Build history of the part. All positions in model axes, mm. A direction names the side the tool comes from. Round coordinates to 2 decimals unless told otherwise and drop trailing zeros. Write each loop counter-clockwise with the first axis right and the second up, starting at its lowest first coordinate (ties: lowest second). Pieces come first, ordered by that corner, then holes. Notation, with made-up numbers: (46.5, 63.5) - (78.5, 63.5) arc R19 ccw to (78.5, 99.5) - close; hole circle Ø7 at (88, -20.5). An arc over 180 degrees is marked (long way). Write each question's results on one line, items separated by ' | '.
from build123d import *

# Parameters (mm, degrees)
F0_W     = 65
F0_H     = 140
F0_W_2   = 9
F0_H_2   = 38
F0_W_3   = 13
F0_H_3   = 14.5
F0_R     = 3.85
F1_DEPTH = 3
F2_DEPTH = 6
F3_DEPTH = 9.5
F4_DEPTH = 13


# Not quite as in the source:
# - a feature names something its author has since deleted; it is built from what else it names


with BuildPart() as f1:
    # F0 (on Top) → F1 (new body)
    with BuildSketch(Plane.XY):
        with Locations((-31.25, -0.0599437952)):
            Rectangle(F0_W, F0_H)
        Polygon((-58.75, -65.0599437952), (-58.75, 64.9400562048), (-3.75, 64.9400562048), (-3.75, 60.4400562048), (-3.75, 49.5400562048), (-3.75, -65.0599437952), align=None, mode=Mode.SUBTRACT)
        Polygon((-3.75, 64.9400562048), (-58.75, 64.9400562048), (-58.75, -65.0599437952), (-3.75, -65.0599437952), (-3.75, 49.5400562048), (-3.75, 60.4400562048), align=None)
        with Locations((-48.45, -37.5599437952)):
            Rectangle(F0_W_2, F0_H_2, mode=Mode.SUBTRACT)
        with Locations((-33.25, -53.8099437952)):
            Rectangle(F0_W_3, F0_H_3, mode=Mode.SUBTRACT)
        with Locations((-33.25, -23.8099437952)):
            Rectangle(F0_W_3, F0_H_3, mode=Mode.SUBTRACT)
        with Locations((-14.75, -38.8099437952)):
            Rectangle(F0_W_3, F0_H_3, mode=Mode.SUBTRACT)
        with Locations((-14.75, -8.8099437952)):
            Rectangle(F0_W_3, F0_H_3, mode=Mode.SUBTRACT)
        with Locations((-48.45, 28.4400562048)):
            Rectangle(F0_W_2, F0_H_2, mode=Mode.SUBTRACT)
        with Locations((-33.25, 6.1900562048)):
            Rectangle(F0_W_3, F0_H_3, mode=Mode.SUBTRACT)
        with Locations((-33.25, 36.1900562048)):
            Rectangle(F0_W_3, F0_H_3, mode=Mode.SUBTRACT)
        with Locations((-14.75, 21.1900562048)):
            Rectangle(F0_W_3, F0_H_3, mode=Mode.SUBTRACT)
        with Locations((-14.75, 51.1900562048)):
            Rectangle(F0_W_3, F0_H_3, mode=Mode.SUBTRACT)
        with Locations((-48.45, 28.4400562048)):
            Rectangle(F0_W_2, F0_H_2)
        with Locations((-48.45, -37.5599437952)):
            Rectangle(F0_W_2, F0_H_2)
        with Locations((-14.75, 51.1900562048)):
            Rectangle(F0_W_3, F0_H_3)
        with Locations((-14.75, 51.1900562048)):
            Circle(F0_R, mode=Mode.SUBTRACT)
        with Locations((-33.25, 36.1900562048)):
            Rectangle(F0_W_3, F0_H_3)
        with Locations((-33.25, 36.1900562048)):
            Circle(F0_R, mode=Mode.SUBTRACT)
        with Locations((-14.75, 21.1900562048)):
            Rectangle(F0_W_3, F0_H_3)
        with Locations((-14.75, 21.1900562048)):
            Circle(F0_R, mode=Mode.SUBTRACT)
        with Locations((-33.25, 6.1900562048)):
            Rectangle(F0_W_3, F0_H_3)
        with Locations((-33.25, 6.1900562048)):
            Circle(F0_R, mode=Mode.SUBTRACT)
        with Locations((-14.75, -8.8099437952)):
            Rectangle(F0_W_3, F0_H_3)
        with Locations((-14.75, -8.8099437952)):
            Circle(F0_R, mode=Mode.SUBTRACT)
        with Locations((-33.25, -23.8099437952)):
            Rectangle(F0_W_3, F0_H_3)
        with Locations((-33.25, -23.8099437952)):
            Circle(F0_R, mode=Mode.SUBTRACT)
        with Locations((-33.25, -53.8099437952)):
            Rectangle(F0_W_3, F0_H_3)
        with Locations((-33.25, -53.8099437952)):
            Circle(F0_R, mode=Mode.SUBTRACT)
        with Locations((-14.75, -38.8099437952)):
            Rectangle(F0_W_3, F0_H_3)
        with Locations((-14.75, -38.8099437952)):
            Circle(F0_R, mode=Mode.SUBTRACT)
    extrude(amount=F1_DEPTH)

    # F0 (on Top) → F2 (join)
    with BuildSketch(Plane.XY):
        with Locations((-31.25, -0.0599437952)):
            Rectangle(F0_W, F0_H)
        Polygon((-58.75, -65.0599437952), (-58.75, 64.9400562048), (-3.75, 64.9400562048), (-3.75, 60.4400562048), (-3.75, 49.5400562048), (-3.75, -65.0599437952), align=None, mode=Mode.SUBTRACT)
        Polygon((-3.75, 64.9400562048), (-58.75, 64.9400562048), (-58.75, -65.0599437952), (-3.75, -65.0599437952), (-3.75, 49.5400562048), (-3.75, 60.4400562048), align=None)
        with Locations((-48.45, -37.5599437952)):
            Rectangle(F0_W_2, F0_H_2, mode=Mode.SUBTRACT)
        with Locations((-33.25, -53.8099437952)):
            Rectangle(F0_W_3, F0_H_3, mode=Mode.SUBTRACT)
        with Locations((-33.25, -23.8099437952)):
            Rectangle(F0_W_3, F0_H_3, mode=Mode.SUBTRACT)
        with Locations((-14.75, -38.8099437952)):
            Rectangle(F0_W_3, F0_H_3, mode=Mode.SUBTRACT)
        with Locations((-14.75, -8.8099437952)):
            Rectangle(F0_W_3, F0_H_3, mode=Mode.SUBTRACT)
        with Locations((-48.45, 28.4400562048)):
            Rectangle(F0_W_2, F0_H_2, mode=Mode.SUBTRACT)
        with Locations((-33.25, 6.1900562048)):
            Rectangle(F0_W_3, F0_H_3, mode=Mode.SUBTRACT)
        with Locations((-33.25, 36.1900562048)):
            Rectangle(F0_W_3, F0_H_3, mode=Mode.SUBTRACT)
        with Locations((-14.75, 21.1900562048)):
            Rectangle(F0_W_3, F0_H_3, mode=Mode.SUBTRACT)
        with Locations((-14.75, 51.1900562048)):
            Rectangle(F0_W_3, F0_H_3, mode=Mode.SUBTRACT)
        with Locations((-48.45, 28.4400562048)):
            Rectangle(F0_W_2, F0_H_2)
        with Locations((-48.45, -37.5599437952)):
            Rectangle(F0_W_2, F0_H_2)
    extrude(amount=F2_DEPTH)

    # F0 (on Top) → F3 (join)
    with BuildSketch(Plane.XY):
        with Locations((-31.25, -0.0599437952)):
            Rectangle(F0_W, F0_H)
        Polygon((-58.75, -65.0599437952), (-58.75, 64.9400562048), (-3.75, 64.9400562048), (-3.75, 60.4400562048), (-3.75, 49.5400562048), (-3.75, -65.0599437952), align=None, mode=Mode.SUBTRACT)
        Polygon((-3.75, 64.9400562048), (-58.75, 64.9400562048), (-58.75, -65.0599437952), (-3.75, -65.0599437952), (-3.75, 49.5400562048), (-3.75, 60.4400562048), align=None)
        with Locations((-48.45, -37.5599437952)):
            Rectangle(F0_W_2, F0_H_2, mode=Mode.SUBTRACT)
        with Locations((-33.25, -53.8099437952)):
            Rectangle(F0_W_3, F0_H_3, mode=Mode.SUBTRACT)
        with Locations((-33.25, -23.8099437952)):
            Rectangle(F0_W_3, F0_H_3, mode=Mode.SUBTRACT)
        with Locations((-14.75, -38.8099437952)):
            Rectangle(F0_W_3, F0_H_3, mode=Mode.SUBTRACT)
        with Locations((-14.75, -8.8099437952)):
            Rectangle(F0_W_3, F0_H_3, mode=Mode.SUBTRACT)
        with Locations((-48.45, 28.4400562048)):
            Rectangle(F0_W_2, F0_H_2, mode=Mode.SUBTRACT)
        with Locations((-33.25, 6.1900562048)):
            Rectangle(F0_W_3, F0_H_3, mode=Mode.SUBTRACT)
        with Locations((-33.25, 36.1900562048)):
            Rectangle(F0_W_3, F0_H_3, mode=Mode.SUBTRACT)
        with Locations((-14.75, 21.1900562048)):
            Rectangle(F0_W_3, F0_H_3, mode=Mode.SUBTRACT)
        with Locations((-14.75, 51.1900562048)):
            Rectangle(F0_W_3, F0_H_3, mode=Mode.SUBTRACT)
    extrude(amount=F3_DEPTH)

    # F0 (on Top) → F4 (join)
    with BuildSketch(Plane.XY):
        with Locations((-31.25, -0.0599437952)):
            Rectangle(F0_W, F0_H)
        Polygon((-58.75, -65.0599437952), (-58.75, 64.9400562048), (-3.75, 64.9400562048), (-3.75, 60.4400562048), (-3.75, 49.5400562048), (-3.75, -65.0599437952), align=None, mode=Mode.SUBTRACT)
    extrude(amount=F4_DEPTH)


solid = f1.part
(1) Slice it at B-B, the plane y = -22. Write the cut outline in (x, z), and give its area (3 significant figures).
Worked answers:
outline: (-63.75, 0) - (-36.65, 0) - (-36.65, 3) - (-39.75, 3) - (-39.75, 9.5) - (-43.95, 9.5) - (-43.95, 6) - (-52.95, 6) - (-52.95, 9.5) - (-58.75, 9.5) - (-58.75, 13) - (-63.75, 13) - close; (-29.85, 0) - (1.25, 0) - (1.25, 13) - (-3.75, 13) - (-3.75, 9.5) - (-26.75, 9.5) - (-26.75, 3) - (-29.85, 3) - close | area: 516 mm2
(2) Slice it at D-D, the plane x = -33.25. State how many separate pieces and enclosed holes the cut face has, and give its area (3 significant figures).
Worked answers:
separate pieces: 5 | enclosed holes: 0 | area: 896 mm2
(3) Tool access for faces 1 (the cylindrical face through (-15.3, 25, 1.5)), 2 (the flat face through (-12, -35, 3)): list every direction of +Z, -Z, +X, -X, +Y, -Y with a clear straight run to the whole face (end or side of a thin tool).
Worked answers:
face 1: +Z, -Z | face 2: +Z
(4) Slice it at A-A, the plane x = -49. Write the cut outline in (y, z), and give its area (3 significant figures).
Worked answers:
outline: (-70.06, 0) - (69.94, 0) - (69.94, 13) - (64.94, 13) - (64.94, 9.5) - (47.44, 9.5) - (47.44, 6) - (9.44, 6) - (9.44, 9.5) - (-18.56, 9.5) - (-18.56, 6) - (-56.56, 6) - (-56.56, 9.5) - (-65.06, 9.5) - (-65.06, 13) - (-70.06, 13) - close | area: 1,100 mm2
(5) Flat gauge pins, fed straight in: pin 1 Ø6 at (x, y) = (-33.25, 6.19) entering from -Z; pin 2 Ø4 at (x, y) = (-30.5, -21) entering from +Z; pin 3 Ø1 at (x, y) = (-39, 20) entering from +Z. Where does each tip first touch, or does it go through?
Worked answers:
pin 1: passes through | pin 2: stops at z = 3 | pin 3: stops at z = 9.5
(6) Drill centre lines: probe 1 along Y at (x, z) = (-33.25, 2.2); probe 2 along Y at (x, z) = (-20.5, 7.5); probe 3 along X at (y, z) = (-27.5, 8.75). Where is each one in solid material? Low to high. Write a range as [from, to].
Worked answers:
probe 1: y = [-70.06, -57.66], [-49.96, -27.66], [-19.96, 2.34], [10.04, 32.34], [40.04, 69.94] | probe 2: y = [-70.06, -46.06], [-31.56, -16.06], [-1.56, 13.94], [28.44, 43.94], [58.44, 69.94] | probe 3: x = [-63.75, -52.95], [-43.95, -39.75], [-26.75, 1.25]
(7) Slice it at C-C, the plane z = 11.5. Write the cut outline in (x, y).
Worked answers:
outline: (-63.75, -70.06) - (1.25, -70.06) - (1.25, 69.94) - (-63.75, 69.94) - close; hole (-58.75, -65.06) - (-3.75, -65.06) - (-3.75, 64.94) - (-58.75, 64.94) - close
(8) Two-plate mould, pull along X, no slides. Class faces 3 (the flat face through (-39.75, 36, 6)), 4 (the flat face through (-32, -70.06, 6)): released by +X, released by -X, zero draft, split by the parting line, or undercut.
Worked answers:
face 3: undercut | face 4: zero draft
